Could you check a few things on this model? Use its own coordinates, in mm. Face numbers are marked on the shaded views. A direction names the side the tool comes from. Coordinates: 2 decimals unless noted, no trailing zeros.
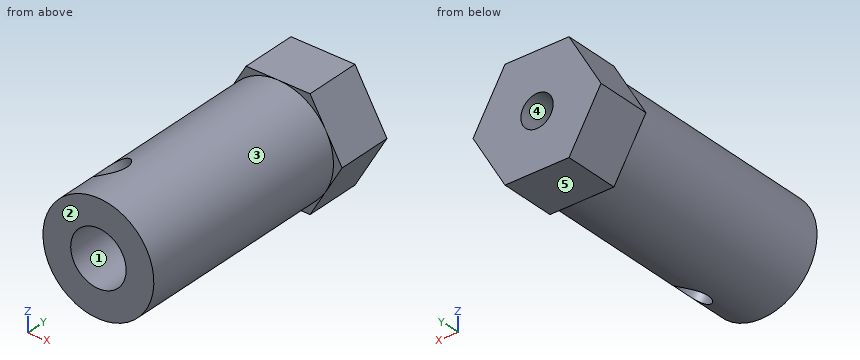
```python
from build123d import *

# Parameters (mm, degrees)
PAD122_DEPTH            = 6
SKETCH186_R             = 6
PAD123_DEPTH            = 24
SKETCH187_R             = 3
POCKET046_DEPTH         = 24.5
SKETCH188_R             = 1.75
POCKET047_DEPTH         = 6
SKETCH189_R             = 1.75
POCKET048_DEPTH         = 7
BODY102_ROLL_ANGLE      = 90.00003
BODY102_PITCH_ANGLE     = -30.000033
BODY102_PLACEMENT_ANGLE = -8e-06


with BuildPart() as part:
    # Sketch185 → Pad122 (new body)
    with BuildSketch(Plane.XY):
        Polygon((6, 3.464102), (0, 6.928203), (-6, 3.464102), (-6, -3.464102), (0, -6.928203), (6, -3.464102), align=None)
    extrude(amount=PAD122_DEPTH)

    # Sketch186 (on Face8 of Pad122) → Pad123 (join)
    with BuildSketch(Plane.XY.offset(6)):
        Circle(SKETCH186_R)
    extrude(amount=PAD123_DEPTH)

    # Sketch187 (on Face15 of Pad123) → Pocket046 (cut)
    with BuildSketch(Plane.XY.offset(30)):
        Circle(SKETCH187_R)
    extrude(amount=-POCKET046_DEPTH, mode=Mode.SUBTRACT)

    # Sketch188 (on Face4 of Pocket046) → Pocket047 (cut)
    with BuildSketch(Plane(origin=(0, 0, 0), x_dir=(1, 0, 0), z_dir=(0, 0, -1))):
        Circle(SKETCH188_R)
    extrude(amount=-POCKET047_DEPTH, mode=Mode.SUBTRACT)

    # Sketch189 → Pocket048 (cut, symmetric)
    with BuildSketch(Plane.XZ):
        with Locations((0, 24.5)):
            Circle(SKETCH189_R)
    extrude(amount=POCKET048_DEPTH, both=True, mode=Mode.SUBTRACT)


with BuildPart() as part_1:
    # Body102 roll: moved
    add(part.part.rotate(Axis((0, 0, 0), (1, 0, 0)), BODY102_ROLL_ANGLE))


with BuildPart() as part_2:
    # Body102 pitch: moved
    add(part_1.part.rotate(Axis((0, 0, 0), (0, 1, 0)), BODY102_PITCH_ANGLE))


with BuildPart() as part_3:
    # Body102 placement: moved
    add(part_2.part.moved(Location((0, 10.3, 0))).rotate(Axis((0, 10.3, 0), (0, 0, 1)), BODY102_PLACEMENT_ANGLE))


solid = part_3.part
```
Item 1: Which directions (+Z, -Z, +X, -X, +Y, -Y) give clear straight access to the entire face, cutting with the end or side of a thin tool? Please do the marked faces 1 and 2.
Item 2: Will these pins go through, and if not, where does the flat tip stop? pin 1 Ø3 at (x, y) = (0.5, -9.5) entering from -Z; pin 2 Ø3 at (x, z) = (0, 0) entering from -Y; pin 3 Ø1.5 at (y, z) = (4, -3.5) entering from -X; pin 4 Ø2 at (y, z) = (-16.5, -0.5) entering from -X.
Item 3: If we mould it in two halves opening along Z, with no side actions, what happens to the marked faces 3, 4 and 5? For each: released by +Z, released by -Z, zero draft, split by the parting line, or undercut.
Item 4: If I drill on line 1 along Y through (x, z) = (2.5, -4); line 2 along Y through (x, z) = (3.75, 4.75); line 3 along Z through (x, y) = (0, -4), over which ranges is the centre line in solid material (lowest first)?
Taken from the geometry:
1. face 1: -Y
1. face 2: +Z, -Z, +X, -X, -Y
2. pin 1: stops at z = -6
2. pin 2: passes through
2. pin 3: stops at x = -5.33
2. pin 4: stops at x = -6
3. face 3: split by the parting line
3. face 4: undercut
3. face 5: released by -Z
4. line 1: y = -19.7 to -15.94, -12.46 to 10.3
4. line 2: y = 4.3 to 10.3
4. line 3: z = -6 to -3, 3 to 6
